Can you work these out from the model? Positions are in its coordinate system, mm. Face numbers are marked on the shaded views. A direction names the side the tool comes from. Give positions to 0.01 mm unless a question says otherwise; leave off trailing zeros. Write each question's results on one line, items separated by ' | '.
from build123d import *

# Parameters (mm, degrees)
SKETCH1_W           = 19.05
SKETCH1_H           = 44.45
SKETCH1_R           = 1.27
BOSS_EXTRUDE1_DEPTH = 9.525
SKETCH2_R           = 2.3622
CUT_EXTRUDE1_DEPTH  = 50.289254661
SKETCH5_R           = 3.175
SKETCH5_R_2         = 2.3622
CUT_EXTRUDE2_DEPTH  = 3.175


with BuildPart() as part:
    # Sketch1 → Boss-Extrude1 (new body)
    with BuildSketch(Plane.XY):
        with Locations((9.525, 22.225)):
            Rectangle(SKETCH1_W, SKETCH1_H)
        with Locations(Location((9.525, 22.225, 0), (0, 0, 180))):
            Circle(SKETCH1_R, mode=Mode.SUBTRACT)
    extrude(amount=BOSS_EXTRUDE1_DEPTH)

    # Sketch2 → Cut-Extrude1 (cut, through all)
    with BuildSketch(Plane(origin=(19.05, 0, 0), x_dir=(0, 0, -1), z_dir=(1, 0, 0))):
        with Locations((-4.7625, 16.51)):
            Circle(SKETCH2_R)
        with Locations((-4.7625, 39.37)):
            Circle(SKETCH2_R)
        with Locations((-4.7625, 27.94)):
            Circle(SKETCH2_R)
        with Locations((-4.7625, 5.08)):
            Circle(SKETCH2_R)
    extrude(amount=-CUT_EXTRUDE1_DEPTH, mode=Mode.SUBTRACT)

    # Sketch5 → Cut-Extrude2 (cut)
    # profile 1 of 4: a face of its own
    with BuildSketch(Plane(origin=(19.05, 0, 0), x_dir=(0, 0, -1), z_dir=(1, 0, 0))):
        with Locations(Location((-4.7625, 5.08, 0), (0, 0, 90))):
            Circle(SKETCH5_R)
        with Locations((-4.7625, 5.08)):
            Circle(SKETCH5_R_2, mode=Mode.SUBTRACT)
    # profile 2 of 4: a face of its own
    with BuildSketch(Plane(origin=(19.05, 0, 0), x_dir=(0, 0, -1), z_dir=(1, 0, 0))):
        with Locations(Location((-4.7625, 16.51, 0), (0, 0, 90))):
            Circle(SKETCH5_R)
        with Locations((-4.7625, 16.51)):
            Circle(SKETCH5_R_2, mode=Mode.SUBTRACT)
    # profile 3 of 4: a face of its own
    with BuildSketch(Plane(origin=(19.05, 0, 0), x_dir=(0, 0, -1), z_dir=(1, 0, 0))):
        with Locations(Location((-4.7625, 27.94, 0), (0, 0, 90))):
            Circle(SKETCH5_R)
        with Locations((-4.7625, 27.94)):
            Circle(SKETCH5_R_2, mode=Mode.SUBTRACT)
    # profile 4 of 4: a face of its own
    with BuildSketch(Plane(origin=(19.05, 0, 0), x_dir=(0, 0, -1), z_dir=(1, 0, 0))):
        with Locations(Location((-4.7625, 39.37, 0), (0, 0, 90))):
            Circle(SKETCH5_R)
        with Locations((-4.7625, 39.37)):
            Circle(SKETCH5_R_2, mode=Mode.SUBTRACT)
    cut_extrude2 = extrude(amount=-CUT_EXTRUDE2_DEPTH, mode=Mode.SUBTRACT)

    # Mirror1: Cut-Extrude2 across plane
    add(cut_extrude2.mirror(Plane(origin=(9.525, 0, 0), x_dir=(0, 0, 1), z_dir=(1, 0, 0))), mode=Mode.SUBTRACT)


solid = part.part
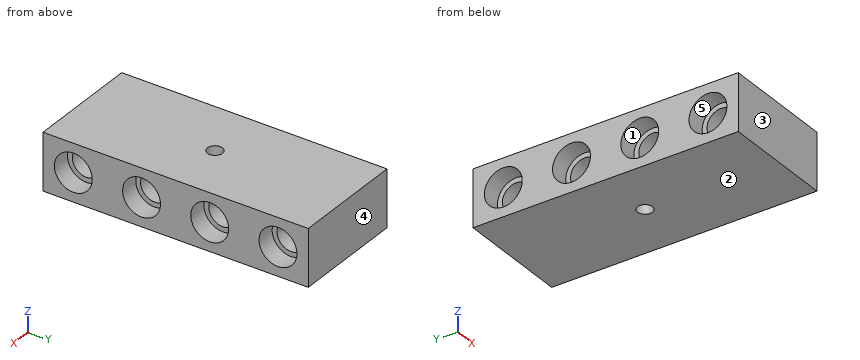
Item 1: I'm going to push flat-ended pins straight in: pin 1 (1.9 mm diameter, centred on y = 26.5, z = 4, fed in from +X) (3 decimals); pin 2 (5.5 mm diameter, centred on y = 27.94, z = 4.76, fed in from -X) (3 decimals); pin 3 (4 mm diameter, centred on y = 16.51, z = 4.76, fed in from +X). Where does each tip first touch, or does it pass through?
Geometry says:
pin 1: stops at x = 15.875 | pin 2: stops at x = 3.175 | pin 3: passes through
Item 2: I want a section at A-A, the plane x = 15. Give the number of separate pieces and of enclosed holes in the cut face, and give its area (3 significant figures).
Geometry says:
separate pieces: 1 | enclosed holes: 4 | area: 353 mm2
Item 3: Thinking about a two-plate mould opening in Y: for the marked faces 3, 4 and 5, which applies, +Y half, -Y half, draft (parallel to the pull), parting line (faces both ways), or undercut?
Geometry says:
face 3: -Y half | face 4: +Y half | face 5: undercut
Item 4: For the marked faces 1 and 2, which set-ups out of +Z, -Z, +X, -X, +Y, -Y let a thin tool reach every point of the face, with its end or its side?
Geometry says:
face 1: -X | face 2: -Z, +X, -X, +Y, -Y
Item 5: If I drill on line 1 (Z direction, x = 0.95, y = 27.94) (1 decimal); line 2 (Y direction, x = 9, z = 5.75); line 3 (Y direction, x = 5, z = 3.5), over which ranges is the centre line in solid material (lowest first)? Write a range as from..to.
Geometry says:
line 1: z = 0..1.6, 7.9..9.5 | line 2: y = 0..2.93, 7.23..14.36, 18.66..21.07, 23.38..25.79, 30.09..37.22, 41.52..44.45 | line 3: y = 0..3.08, 7.08..14.51, 18.51..25.94, 29.94..37.37, 41.37..44.45
